Design review of the part built by this model. Coordinates are the model's own, in mm. A direction names the side the tool comes from. Give positions to 0.01 mm unless a question says otherwise; leave off trailing zeros. Loops run counter-clockwise (first coordinate to the right, second up) from the corner with the lowest first, then second, coordinate; pieces in that order, holes last.
from build123d import *

# Parameters (mm, degrees)
SKETCH1_W                              = 209
SKETCH1_H                              = 239
BASE_PLATE_DEPTH                       = 4
MOUNTING_HOLES_START                   = 1.5
MOUNTING_HOLES_OUTLINE_R               = 3.25
MOUNTING_HOLES_DEPTH                   = 2.5
MOUNTING_HOLES_2_OUTLINE_R             = 1.7
MOUNTING_HOLES_2_DEPTH                 = 1.5
MOUNTING_HOLES_MIRROR2_START           = 1.5
MOUNTING_HOLES_MIRROR2_COPY_1_SKETCH_R = 3.25
MOUNTING_HOLES_MIRROR2_COPY_1_DEPTH    = 2.5
MOUNTING_HOLES_MIRROR2_COPY_2_SKETCH_R = 1.7
MOUNTING_HOLES_MIRROR2_COPY_2_DEPTH    = 1.5
MOUNTING_HOLES_MIRROR2_COPY_3_SKETCH_R = 1.7
MOUNTING_HOLES_MIRROR2_COPY_3_DEPTH    = 1.5
SKETCH5_W                              = 129
SKETCH5_H                              = 4
SIDE_EXTRUSION_DEPTH                   = 14
SKETCH6_W                              = 4
SKETCH6_H                              = 164
UPPER_LOWER_EXTRUSION_DEPTH            = 14
EDGE_FILLETS_R                         = 3


# Read off the part's stored shape, not the designer's step: mounting_holes
with BuildPart() as part:
    # Sketch1 → base_plate (new body)
    with BuildSketch(Plane(origin=(0, 0, 0), x_dir=(1, 0, 0), z_dir=(0, 1, 0))):
        Rectangle(SKETCH1_W, SKETCH1_H)
    extrude(amount=BASE_PLATE_DEPTH)

    # mounting_holes outline → mounting_holes (cut)
    with BuildSketch(Plane(origin=(0, 0, 0), x_dir=(1, 0, 0), z_dir=(0, 1, 0)).offset(MOUNTING_HOLES_START)):
        with Locations((95, 95)):
            Circle(MOUNTING_HOLES_OUTLINE_R)
        with Locations((80, 110)):
            Circle(MOUNTING_HOLES_OUTLINE_R)
    mounting_holes = extrude(amount=MOUNTING_HOLES_DEPTH, mode=Mode.SUBTRACT)

    # mounting_holes 2 outline → mounting_holes 2 (cut)
    with BuildSketch(Plane(origin=(0, 0, 0), x_dir=(1, 0, 0), z_dir=(0, 1, 0))):
        with Locations((95, 95)):
            Circle(MOUNTING_HOLES_2_OUTLINE_R)
        with Locations((80, 110)):
            Circle(MOUNTING_HOLES_2_OUTLINE_R)
    mounting_holes_2 = extrude(amount=MOUNTING_HOLES_2_DEPTH, mode=Mode.SUBTRACT)

    # mounting_holes_mirror1: mounting_holes, mounting_holes 2 across plane
    add(mounting_holes.mirror(Plane.XY), mode=Mode.SUBTRACT)
    add(mounting_holes_2.mirror(Plane.XY), mode=Mode.SUBTRACT)

    # mounting_holes_mirror2: mounting_holes, mounting_holes 2 across plane
    add(mounting_holes.mirror(Plane(origin=(0, 0, 0), x_dir=(0, 0, 1), z_dir=(1, 0, 0))), mode=Mode.SUBTRACT)
    add(mounting_holes_2.mirror(Plane(origin=(0, 0, 0), x_dir=(0, 0, 1), z_dir=(1, 0, 0))), mode=Mode.SUBTRACT)

    # mounting_holes_mirror2 copy 1 sketch → mounting_holes_mirror2 copy 1 (cut)
    with BuildSketch(Plane(origin=(0, 0, 0), x_dir=(-1, 0, 0), z_dir=(0, 1, 0)).offset(MOUNTING_HOLES_MIRROR2_START)):
        with Locations((95, 95)):
            Circle(MOUNTING_HOLES_MIRROR2_COPY_1_SKETCH_R)
        with Locations((80, 110)):
            Circle(MOUNTING_HOLES_MIRROR2_COPY_1_SKETCH_R)
    extrude(amount=MOUNTING_HOLES_MIRROR2_COPY_1_DEPTH, mode=Mode.SUBTRACT)

    # mounting_holes_mirror2 copy 2 sketch → mounting_holes_mirror2 copy 2 (cut)
    with BuildSketch(Plane(origin=(0, 0, 0), x_dir=(-1, 0, 0), z_dir=(0, 1, 0))):
        with Locations((95, 95)):
            Circle(MOUNTING_HOLES_MIRROR2_COPY_2_SKETCH_R)
        with Locations((80, 110)):
            Circle(MOUNTING_HOLES_MIRROR2_COPY_2_SKETCH_R)
    extrude(amount=MOUNTING_HOLES_MIRROR2_COPY_2_DEPTH, mode=Mode.SUBTRACT)

    # mounting_holes_mirror2 copy 3 sketch → mounting_holes_mirror2 copy 3 (cut)
    with BuildSketch(Plane(origin=(0, 0, 0), x_dir=(-1, 0, 0), z_dir=(0, 1, 0))):
        with Locations((95, -95)):
            Circle(MOUNTING_HOLES_MIRROR2_COPY_3_SKETCH_R)
        with Locations((80, -110)):
            Circle(MOUNTING_HOLES_MIRROR2_COPY_3_SKETCH_R)
    extrude(amount=MOUNTING_HOLES_MIRROR2_COPY_3_DEPTH, mode=Mode.SUBTRACT)

    # Sketch5 → side_extrusion (add)
    with BuildSketch(Plane(origin=(0, 4, 0), x_dir=(1, 0, 0), z_dir=(0, 1, 0))):
        with Locations((0, 121.5)):
            Rectangle(SKETCH5_W, SKETCH5_H)
    extrude(amount=-SIDE_EXTRUSION_DEPTH)

    # Sketch6 → upper_lower_extrusion (add)
    with BuildSketch(Plane(origin=(0, 4, 0), x_dir=(1, 0, 0), z_dir=(0, 1, 0))):
        with Locations((-106.5, -2.5)):
            Rectangle(SKETCH6_W, SKETCH6_H)
        with Locations((106.5, -2.5)):
            Rectangle(SKETCH6_W, SKETCH6_H)
    extrude(amount=-UPPER_LOWER_EXTRUSION_DEPTH)

    # edge_fillets
    edge_fillets_edges = [part.edges().sort_by_distance(p)[0] for p in [
        (104.5, 2, 119.5),
        (-104.5, 2, 119.5),
        (-104.5, 2, -119.5),
        (104.5, 2, -119.5),
    ]]
    fillet(edge_fillets_edges, radius=EDGE_FILLETS_R)


solid = part.part
Q1. Take a section at B-B (z = -18.5). Give the boundary of the cut face in (x, y).
Results:
outline: (-108.5, -10) - (-104.5, -10) - (-104.5, 0) - (104.5, 0) - (104.5, -10) - (108.5, -10) - (108.5, 4) - (-108.5, 4) - close
Q2. Take a section at A-A (y = -7.75). Give the boundary of the cut face in (x, z), plus the area to 3 significant figures.
Results:
outline: (-108.5, -79.5) - (-104.5, -79.5) - (-104.5, 84.5) - (-108.5, 84.5) - close; (-64.5, -123.5) - (64.5, -123.5) - (64.5, -119.5) - (-64.5, -119.5) - close; (104.5, -79.5) - (108.5, -79.5) - (108.5, 84.5) - (104.5, 84.5) - close
area: 1,830 mm2
Q3. Draft analysis for pull direction X (two halves, no side actions). For faces 1 (the face through (79.295, 2.732, 106.827)), 2 (the face through (108.5, -3, 4)), 3 (the face through (-1, -3, -123.5)), state which applies: pulls with the +X half, pulls with the -X half, needs draft (parallel to the pull), parting line crosses it, or undercut.
Results:
face 1: undercut
face 2: pulls with the +X half
face 3: needs draft
Q4. Insertion check: pin 1 (4 mm diameter, centred on x = 14.5, z = 69, fed in from -Y); pin 2 (5 mm diameter, centred on x = -95.5, z = -95.5, fed in from +Y); pin 3 (1.2 mm diameter, centred on y = 2, z = 101.5, fed in from +X); pin 4 (7.5 mm diameter, centred on x = -95, z = 95, fed in from +Y). Each pin has a flat end and moves straight along its axis. Give the tip position at first contact, or say it passes through.
Results:
pin 1: stops at y = 0
pin 2: stops at y = 1.5
pin 3: stops at x = 104.5
pin 4: stops at y = 4
Q5. Tool access review of faces 4 (the face through (-94.295, 2.732, -91.827)), 5 (the face through (-1, 0, -2)), 6 (the face through (-2, 4, -4)), 7 (the face through (-108.5, -3, 4)), 8 (the face through (104.5, -5, 4)): name each direction out of +Z, -Z, +X, -X, +Y, -Y from which nothing blocks a thin tool from reaching the whole face with its end or side.
Results:
face 4: +Y
face 5: +Z, -Y
face 6: +Z, -Z, +X, -X, +Y
face 7: +Z, -Z, -X, +Y, -Y
face 8: +Z, -Z, -Y
Q6. Wall thickness on line 1 (X direction, y = 2.1, z = -95); line 2 (Z direction, x = 95, y = 3); line 3 (X direction, y = 0.4, z = -110): over which ranges is each line inside the solid? List them lowest first.
Results:
line 1: x = -104.5 to -98.25, -91.75 to 91.75, 98.25 to 104.5
line 2: z = -119.5 to -98.25, -91.75 to 91.75, 98.25 to 119.5
line 3: x = -104.5 to -81.7, -78.3 to 78.3, 81.7 to 104.5
Q7. Take a section at D-D (x = -69.5). Give the boundary of the cut face in (y, z), plus the area to 3 significant figures.
Results:
outline: (0, -119.5) - (4, -119.5) - (4, 119.5) - (0, 119.5) - close
area: 956 mm2
Q8. Take a section at C-C (x = 17). Give the boundary of the cut face in (y, z), plus the area to 3 significant figures.
Results:
outline: (-10, -123.5) - (4, -123.5) - (4, 119.5) - (0, 119.5) - (0, -119.5) - (-10, -119.5) - close
area: 1,010 mm2
